Check sheet for the modelled part. Datum: model origin and axes. Units: mm. Face numbers are marked on the shaded views. A direction names the side the tool comes from. Coordinates: 2 decimals unless noted, no trailing zeros. Loops run counter-clockwise (first coordinate to the right, second up) from the corner with the lowest first, then second, coordinate; pieces in that order, holes last. Notation, with made-up numbers: M 9.25,-12 L 57.25,-12 A18 cw 57.25,11 Z; hole C -27,67 d9. An arc over 180 degrees is marked long. Return JSON: item names as keys, results as strings.
from build123d import *
from build123d.topology import SkipClean

# Parameters (mm, degrees)
SKETCH_1_R                            = 17
SKETCH_1_R_2                          = 12
EXTRUDE_2_DEPTH                       = 35
SKETCH_3_W                            = 33.795275063
SKETCH_3_H                            = 34.72803434
SKETCH_3_R                            = 13
EXTRUDE_7_DEPTH                       = 45
SKETCH_4_R                            = 13
CUT_EXTRUDE_1_DEPTH                   = 60.489495005
SKETCH_12_R                           = 2
CUT_EXTRUDE_11_DEPTH                  = 45
SKETCH_15_R                           = 2
CUT_EXTRUDE_12_DEPTH                  = 45
FILLET_4_R                            = 10
SKETCH_20_R                           = 13
CUT_EXTRUDE_18_DEPTH                  = 31
EXTRUDE_START                         = 1
SKETCH_25_R                           = 13
EXTRUDE_10_DEPTH                      = 1
CUT_EXTRUDE_19_REACH                  = 68.273
CUT_EXTRUDE_19_END_RADIUS             = 13
SKETCH_26_W                           = 35
SKETCH_26_H                           = 2
CUT_EXTRUDE_19_DIRECTION_2_REACH      = 68.273
CUT_EXTRUDE_19_DIRECTION_2_END_RADIUS = 17
EXTRUDE_11_DEPTH                      = 12
EXTRUDE_11_DEPTH_BACK                 = 3
SKETCH_27_W                           = 14.7
SKETCH_27_H                           = 7.5
EXTRUDE_12_DEPTH                      = 5
SKETCH_30_R                           = 1.6
CUT_EXTRUDE_21_DEPTH                  = 5
CUT_EXTRUDE_22_DEPTH                  = 3.2
SKETCH_34_R                           = 2
CUT_EXTRUDE_23_DEPTH                  = 59.192936687


with BuildPart() as part:
    # Эскиз1 → Бобышка-Вытянуть2 (new body)
    with BuildSketch(Plane.XY):
        Circle(SKETCH_1_R)
        Circle(SKETCH_1_R_2, mode=Mode.SUBTRACT)
    extrude(amount=EXTRUDE_2_DEPTH)

    # Эскиз3 → Бобышка-Вытянуть7 (add)
    with BuildSketch(Plane(origin=(0, 45, 0), x_dir=(1, 0, 0), z_dir=(0, 1, 0))):
        with Locations((0.102362468, -17.511098906)):
            Rectangle(SKETCH_3_W, SKETCH_3_H)
        with Locations(Location((0, -17.5, 0), (0, 0, 270))):
            Circle(SKETCH_3_R, mode=Mode.SUBTRACT)
    extrude(amount=-EXTRUDE_7_DEPTH)

    # Эскиз4 → Вырез-Вытянуть1 (cut, through all)
    with BuildSketch(Plane(origin=(0, 0, 0), x_dir=(-1, 0, 0), z_dir=(0, 0, -1))):
        Circle(SKETCH_4_R)
    extrude(amount=-CUT_EXTRUDE_1_DEPTH, mode=Mode.SUBTRACT)

    # Эскиз12 → Вырез-Вытянуть11 (cut)
    with BuildSketch(Plane(origin=(0, 0, 0), x_dir=(-1, 0, 0), z_dir=(0, 0, -1))):
        with Locations((0, 23)):
            Circle(SKETCH_12_R)
    extrude(amount=-CUT_EXTRUDE_11_DEPTH, mode=Mode.SUBTRACT)

    # Эскиз15 → Вырез-Вытянуть12 (cut)
    with BuildSketch(Plane.ZY.offset(16.795275063)):
        with Locations((17.5, 33)):
            Circle(SKETCH_15_R)
    extrude(amount=-CUT_EXTRUDE_12_DEPTH, mode=Mode.SUBTRACT)

    # Скругление4
    # the kernel refuses this fillet: 10 mm, written as the material it takes off along each edge
    with BuildSketch(Plane(origin=(-16.795275063, 70, 34.875116076), x_dir=(1, 0, 0), z_dir=(0, -1, 0))) as fillet_4_piece_1_section:
        with BuildLine():
            CenterArc((FILLET_4_R, -FILLET_4_R), FILLET_4_R, 90, 90)
            Line((0, -FILLET_4_R), (0, 0))
            Line((0, 0), (FILLET_4_R, 0))
        make_face()
    fillet_4_piece_1 = extrude(amount=92.369651061, mode=Mode.PRIVATE)
    fillet_4_piece_1 = fillet_4_piece_1 - Plane(origin=(0, 0, 32.54483178), x_dir=(1, 0, 0), z_dir=(0, 0, -1)) * Cylinder(17, 225, mode=Mode.PRIVATE)
    add(fillet_4_piece_1, mode=Mode.SUBTRACT)
    with BuildSketch(Plane(origin=(17, 70, 0.147081736), x_dir=(0, 0, 1), z_dir=(0, -1, 0))) as fillet_4_piece_2_section:
        with BuildLine():
            CenterArc((FILLET_4_R, FILLET_4_R), FILLET_4_R, 180, 90)
            Line((0, FILLET_4_R), (0, 0))
            Line((0, 0), (FILLET_4_R, 0))
        make_face()
    fillet_4_piece_2 = extrude(amount=95, mode=Mode.PRIVATE)
    fillet_4_piece_2 = fillet_4_piece_2 - Plane(origin=(0, 0, 2.486350956), x_dir=(1, 0, 0), z_dir=(0, 0, -1)) * Cylinder(17, 230, mode=Mode.PRIVATE)
    add(fillet_4_piece_2, mode=Mode.SUBTRACT)
    with BuildSketch(Plane(origin=(17, 70, 34.875116076), x_dir=(0, 0, -1), z_dir=(0, -1, 0))) as fillet_4_piece_3_section:
        with BuildLine():
            CenterArc((FILLET_4_R, -FILLET_4_R), FILLET_4_R, 90, 90)
            Line((0, -FILLET_4_R), (0, 0))
            Line((0, 0), (FILLET_4_R, 0))
        make_face()
    fillet_4_piece_3 = extrude(amount=95, mode=Mode.PRIVATE)
    fillet_4_piece_3 = fillet_4_piece_3 - Plane(origin=(0, 0, 32.535846855), x_dir=(1, 0, 0), z_dir=(0, 0, -1)) * Cylinder(17, 230, mode=Mode.PRIVATE)
    add(fillet_4_piece_3, mode=Mode.SUBTRACT)
    with BuildSketch(Plane(origin=(-16.795275063, 70, 0.147081736), x_dir=(0, 0, 1), z_dir=(0, -1, 0))) as fillet_4_piece_4_section:
        with BuildLine():
            CenterArc((FILLET_4_R, -FILLET_4_R), FILLET_4_R, 90, 90)
            Line((0, -FILLET_4_R), (0, 0))
            Line((0, 0), (FILLET_4_R, 0))
        make_face()
    fillet_4_piece_4 = extrude(amount=92.369651061, mode=Mode.PRIVATE)
    fillet_4_piece_4 = fillet_4_piece_4 - Plane(origin=(0, 0, 2.477367304), x_dir=(1, 0, 0), z_dir=(0, 0, -1)) * Cylinder(17, 225, mode=Mode.PRIVATE)
    add(fillet_4_piece_4, mode=Mode.SUBTRACT)

    # Эскиз20 → Вырез-Вытянуть18 (cut)
    with SkipClean():  # the faces are left unmerged after this step: merging them gives an invalid solid
        with BuildSketch(Plane(origin=(0, 45, 0), x_dir=(1, 0, 0), z_dir=(0, 1, 0))):
            with Locations(Location((0, -17.5, 0), (0, 0, 270))):
                Circle(SKETCH_20_R)
        extrude(amount=-CUT_EXTRUDE_18_DEPTH, mode=Mode.SUBTRACT)

    # Эскиз25 → Бобышка-Вытянуть10 (add)
    with BuildSketch(Plane(origin=(0, 14, 0), x_dir=(1, 0, 0), z_dir=(0, 1, 0)).offset(EXTRUDE_START)):
        with Locations(Location((0, -17.5, 0), (0, 0, 270))):
            Circle(SKETCH_25_R)
    extrude(amount=-EXTRUDE_10_DEPTH)

    # Вырез-Вытянуть19: up to this cylinder (the profile starts outside it)
    cut_extrude_19_end = Plane(origin=(0, 0, 17.5), z_dir=(0, 0, -1)) * Cylinder(CUT_EXTRUDE_19_END_RADIUS, 163.546, mode=Mode.PRIVATE)
    # Эскиз26 → Вырез-Вытянуть19 (cut, up to the surface)
    with BuildSketch(Plane.ZY.offset(16.795275063), mode=Mode.PRIVATE) as cut_extrude_19_sk1:
        with Locations((17.5, 0)):
            Rectangle(SKETCH_26_W, SKETCH_26_H)
    cut_extrude_19_tool1 = extrude(cut_extrude_19_sk1.sketch, amount=-CUT_EXTRUDE_19_REACH, mode=Mode.PRIVATE) - cut_extrude_19_end
    add(cut_extrude_19_tool1.solids().sort_by_distance((-16.795275, 0, 17.5))[0], mode=Mode.SUBTRACT)

    # Вырез-Вытянуть19 direction 2: up to this cylinder (the profile starts inside it)
    cut_extrude_19_direction_2_end = Plane(origin=(0, 0, 17.5), z_dir=(0, 0, -1)) * Cylinder(CUT_EXTRUDE_19_DIRECTION_2_END_RADIUS, 171.546, mode=Mode.PRIVATE)
    # Эскиз26 → Вырез-Вытянуть19 direction 2 (cut, up to the surface)
    with BuildSketch(Plane.ZY.offset(16.795275063), mode=Mode.PRIVATE) as cut_extrude_19_direction_2_sk1:
        with Locations((17.5, 0)):
            Rectangle(SKETCH_26_W, SKETCH_26_H)
    cut_extrude_19_direction_2_tool1 = extrude(cut_extrude_19_direction_2_sk1.sketch, amount=CUT_EXTRUDE_19_DIRECTION_2_REACH, mode=Mode.PRIVATE) & cut_extrude_19_direction_2_end
    add(cut_extrude_19_direction_2_tool1.solids().sort_by_distance((-16.795275, 0, 17.5))[0], mode=Mode.SUBTRACT)

    # Эскиз27 → Бобышка-Вытянуть11 (add, two sides: drawn at the far end of the back side and taken through both)
    with BuildSketch(Plane.ZY.offset(16.795275063).offset(-EXTRUDE_11_DEPTH_BACK)):
        with Locations((17.497081736, 4.75)):
            Rectangle(SKETCH_27_W, SKETCH_27_H)
        with Locations((17.497081736, -4.75)):
            Rectangle(SKETCH_27_W, SKETCH_27_H)
    extrude(amount=EXTRUDE_11_DEPTH + EXTRUDE_11_DEPTH_BACK)

    # Эскиз29 → Бобышка-Вытянуть12 (add)
    with BuildSketch(Plane(origin=(0, 0, 0), x_dir=(-1, 0, 0), z_dir=(0, 0, -1))):
        with BuildLine():
            Line((3.04805277, -12.647504667), (3.04805277, -3.334582187))
            ThreePointArc((3.04805277, -3.334582187), (-4.517749888, 0), (3.04805277, 3.334582187))
            Line((3.04805277, 3.334582187), (3.04805277, 12.647504667))
            ThreePointArc((3.04805277, 12.647504667), (-13.009611831, 0), (3.04805277, -12.647504667))
        make_face()
    extrude(amount=-EXTRUDE_12_DEPTH)

    # Эскиз30 → Вырез-Вытянуть21 (cut)
    with BuildSketch(Plane(origin=(0, 0, 0), x_dir=(-1, 0, 0), z_dir=(0, 0, -1))):
        with Locations((-0.517749888, -8.75)):
            Circle(SKETCH_30_R)
        with Locations((-0.517749888, 8.75)):
            Circle(SKETCH_30_R)
    extrude(amount=-CUT_EXTRUDE_21_DEPTH, mode=Mode.SUBTRACT)

    # Эскиз28 → Вырез-Вытянуть22 (cut)
    with BuildSketch(Plane(origin=(0, 8.5, 0), x_dir=(1, 0, 0), z_dir=(0, 1, 0))):
        Polygon((-25.595275063, -17.497081736), (-24.195275063, -19.921952866), (-21.395275063, -19.921952866), (-19.995275063, -17.497081736), (-21.395275063, -15.072210605), (-24.195275063, -15.072210605), align=None)
    extrude(amount=-CUT_EXTRUDE_22_DEPTH, mode=Mode.SUBTRACT)

    # Эскиз34 → Вырез-Вытянуть23 (cut, through all)
    with BuildSketch(Plane(origin=(0, 8.5, 0), x_dir=(1, 0, 0), z_dir=(0, 1, 0))):
        with Locations(Location((-22.795275063, -17.497081736, 0), (0, 0, 270))):
            Circle(SKETCH_34_R)
    extrude(amount=-CUT_EXTRUDE_23_DEPTH, mode=Mode.SUBTRACT)


solid = part.part
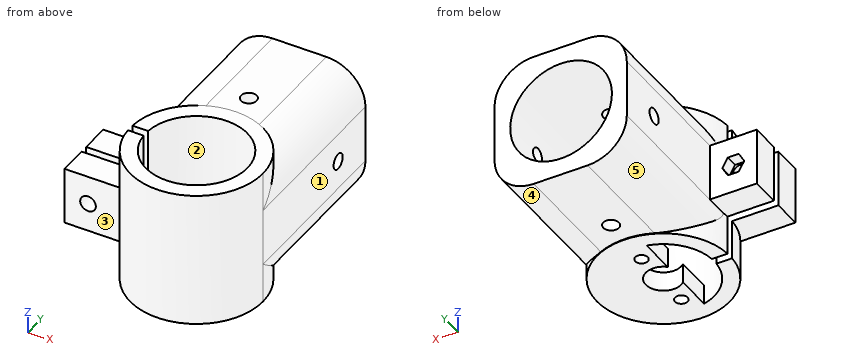
1) Go/stop test with flat-tipped pins: pin 1 Ø6.5 at (x, y) = (0, 23) entering from -Z; pin 2 Ø5 at (x, z) = (1.5, 17.5) entering from -Y; pin 3 Ø2.5 at (x, z) = (-21.5, 18.5) entering from +Y; pin 4 Ø1 at (x, z) = (-11, 17.5) entering from -Y. Record where each tip stops, or that it passes through.
Answers:
{"pin 1": "z = 0.15", "pin 2": "y = -17", "pin 3": "y = 8.5", "pin 4": "y = -13.37"}
2) Section check C-C on y = 33. Record the cut outline in (x, z), then the cut area to 3 significant figures.
Answers:
{"outline": "M -16.8,10.15 A10 ccw -6.8,0.15 L 7,0.15 A10 ccw 17,10.15 L 17,15.5 L 12.85,15.5 A13 cw -12.85,15.5 L -16.8,15.5 Z; M -16.8,19.5 L -12.85,19.5 A13 cw 12.85,19.5 L 17,19.5 L 17,24.88 A10 ccw 7,34.88 L -6.8,34.88 A10 ccw -16.8,24.88 Z", "area": "525 mm²"}
3) Scan lines: line 1 along Y through (x, z) = (-18, 23); line 2 along Y through (x, z) = (0, 31); line 3 along Y through (x, z) = (-15, 31). Record each from-to range of solid material in increasing order. Write a range as [from, to].
Answers:
{"line 1": "[-8.5, -1], [1, 8.5]", "line 2": "[-17, -13], [13, 21], [25, 45]", "line 3": "[-8, -1], [1, 8]"}
4) Set-up check for the marked faces 4 and 5: record each of +Z, -Z, +X, -X, +Y, -Y from which the full face is reachable in a straight line by a thin tool's end or side.
Answers:
{"face 4": "-Z, +X, +Y", "face 5": "-Z, -X, +Y"}
5) Section check D-D on y = 40. Record the cut outline in (x, z).
Answers:
{"outline": "M -16.8,10.15 A10 ccw -6.8,0.15 L 7,0.15 A10 ccw 17,10.15 L 17,24.88 A10 ccw 7,34.88 L -6.8,34.88 A10 ccw -16.8,24.88 Z; hole C 0,17.5 d26"}
6) Section check A-A on y = -6. Record the cut outline in (x, z), then the cut area to 3 significant figures.
Answers:
{"outline": "M -28.8,10.15 L -15.91,10.15 L -15.91,0 L -11.53,0 L -11.53,35 L -15.91,35 L -15.91,24.85 L -28.8,24.85 Z; M -3.05,0 L 15.91,0 L 15.91,35 L 11.53,35 L 11.53,5 L -3.05,5 Z; hole C -22.8,17.5 d4", "area": "556 mm²"}
7) Draft check along X on the marked faces 1, 2 and 3. Enter one of: +X half, -X half, draft (parallel to the pull), parting line (faces both ways), or undercut.
Answers:
{"face 1": "+X half", "face 2": "undercut", "face 3": "draft"}
8) Section check B-B on x = 3. Record the cut outline in (y, z).
Answers:
{"outline": "M -16.73,0 L -3.38,0 L -3.38,5 L -12.65,5 L -12.65,35 L -16.73,35 Z; M 3.38,0 L 16.73,0 L 16.73,0.15 L 45,0.15 L 45,4.85 L 15,4.85 L 15,30.15 L 45,30.15 L 45,34.88 L 16.73,34.88 L 16.73,35 L 12.65,35 L 12.65,5 L 3.38,5 Z"}
